The model under review builds one solid part; all positions refer to its coordinate system, in mm. Face numbers are marked on the shaded views. A direction names the side the tool comes from. Round coordinates to 2 decimals unless told otherwise and drop trailing zeros. Order: outer loops, then holes, each group sorted by start corner. A loop starts at its lowest first (then second) coordinate and runs counter-clockwise, first axis right, second up. Notation, with made-up numbers: M 80,64 L 124,64 A19 cw 124,78 Z; hole C 0.25,-28 d3. An arc over 180 degrees is marked long. Use a Markdown table: item, result. Add a question column.
1. Consider section B-B on x = 41.8. State the section outline as (y, z) points.
2. Consider section D-D on z = 17. State the section outline as (x, y) points.
3. To check wall thickness, follow probe 1 along X at (y, z) = (11.5, 12); probe 2 along Z at (x, y) = (11.5, 38); probe 3 along Z at (x, y) = (41.8, 12.6). State the ranges of each line that lie inside material, in increasing order.
4. The part is to be moulded in two halves that separate along X. For the marked faces 3, 4 and 5, say which applies: +X half, -X half, draft (parallel to the pull), parting line (faces both ways), or undercut.
5. Consider section A-A on y = 11. State the section outline as (x, z) points, then the cut area to 3 significant figures.
6. Consider section C-C on y = 23.5. State the section outline as (x, z) points.
7. Insertion check: P1, Ø1.2, axis at x = 50, z = 0, coming from the +Y side; P2, Ø2.5, axis at x = 8, z = 7.5, coming from the +Y side; P3, Ø0.8, axis at x = 41.5, z = 23.5, coming from the +Y side. Each pin has a flat end and moves straight along its axis. Give the tip position at first contact, or say it passes through.
8. For the marked faces 1 and 2, list the 3-axis set-ups (+Z, -Z, +X, -X, +Y, -Y) from which the entire face can be reached by the end or side of a thin tool; tool diameter is ignored.
from build123d import *

# Parameters (mm, degrees)
SKETCH1_W           = 50
SKETCH1_H           = 30
BOSS_EXTRUDE1_DEPTH = 5
SKETCH1_3_W         = 60
SKETCH1_3_H         = 40
SKETCH1_3_W_2       = 50
SKETCH1_3_H_2       = 30
BOSS_EXTRUDE2_DEPTH = 40
SKETCH2_R           = 4
BOSS_EXTRUDE3_DEPTH = 10
SKETCH6_R           = 0.75
CUT_EXTRUDE1_DEPTH  = 5
FILLET1_R           = 1.5
BOSS_EXTRUDE4_START = -1e-06
BOSS_EXTRUDE4_DEPTH = 35.000001
SKETCH10_R          = 0.75
CUT_EXTRUDE2_DEPTH  = 10
FILLET2_R           = 1


with BuildPart() as part:
    # Sketch1 → Boss-Extrude1 (new body)
    with BuildSketch(Plane(origin=(0, 0, 0), x_dir=(1, 0, 0), z_dir=(0, 1, 0))):
        with Locations((25, -15)):
            Rectangle(SKETCH1_W, SKETCH1_H)
    extrude(amount=BOSS_EXTRUDE1_DEPTH)

    # Sketch1<3> → Boss-Extrude2 (add)
    with BuildSketch(Plane(origin=(0, 0, 0), x_dir=(1, 0, 0), z_dir=(0, 1, 0))):
        with Locations((25, -15)):
            Rectangle(SKETCH1_3_W, SKETCH1_3_H)
        with Locations((25, -15)):
            Rectangle(SKETCH1_3_W_2, SKETCH1_3_H_2, mode=Mode.SUBTRACT)
    extrude(amount=BOSS_EXTRUDE2_DEPTH)

    # Sketch2 → Boss-Extrude3 (add)
    with BuildSketch(Plane(origin=(0, 5, 0), x_dir=(1, 0, 0), z_dir=(0, 1, 0))):
        with Locations((8.2, -6.5)):
            Circle(SKETCH2_R)
        with Locations((41.8, -23.5)):
            Circle(SKETCH2_R)
    extrude(amount=BOSS_EXTRUDE3_DEPTH)

    # Sketch6 → Cut-Extrude1 (cut)
    with BuildSketch(Plane(origin=(0, 15, 0), x_dir=(1, 0, 0), z_dir=(0, 1, 0))):
        with Locations((41.8, -23.4)):
            Circle(SKETCH6_R)
        with Locations((8.1, -6.6)):
            Circle(SKETCH6_R)
    extrude(amount=-CUT_EXTRUDE1_DEPTH, mode=Mode.SUBTRACT)

    # Fillet1
    fillet1_edges = [part.edges().sort_by_distance(p)[0] for p in [
        (4.2, 5, 6.5),
        (37.8, 5, 23.5),
    ]]
    fillet(fillet1_edges, radius=FILLET1_R)

    # Sketch9 → Boss-Extrude4 (add)
    with BuildSketch(Plane(origin=(0, 5, 0), x_dir=(1, 0, 0), z_dir=(0, 1, 0)).offset(BOSS_EXTRUDE4_START)):
        with BuildLine():
            Line((5, 0), (0, 0))
            Line((0, 0), (0, -5))
            ThreePointArc((0, -5), (3.535533906, -3.535533906), (5, 0))
        make_face()
        with BuildLine():
            Line((50, -5), (50, 0))
            Line((50, 0), (45, 0))
            ThreePointArc((45, 0), (46.464466094, -3.535533906), (50, -5))
        make_face()
        with BuildLine():
            Line((45, -30), (50, -30))
            Line((50, -30), (50, -25))
            ThreePointArc((50, -25), (46.464466094, -26.464466094), (45, -30))
        make_face()
        with BuildLine():
            Line((0, -25), (0, -30))
            Line((0, -30), (5, -30))
            ThreePointArc((5, -30), (3.535533906, -26.464466094), (0, -25))
        make_face()
    extrude(amount=BOSS_EXTRUDE4_DEPTH)

    # Sketch10 → Cut-Extrude2 (cut)
    with BuildSketch(Plane(origin=(0, 40, 0), x_dir=(1, 0, 0), z_dir=(0, 1, 0))):
        with Locations((50, -30)):
            Circle(SKETCH10_R)
        with Locations((0, -30)):
            Circle(SKETCH10_R)
        with Locations((50, 0)):
            Circle(SKETCH10_R)
        Circle(SKETCH10_R)
    extrude(amount=-CUT_EXTRUDE2_DEPTH, mode=Mode.SUBTRACT)

    # Fillet2
    fillet2_edges = [part.edges().sort_by_distance(p)[0] for p in [
        (-5, 20, -5),
        (-5, 20, 35),
        (55, 20, 35),
        (55, 20, -5),
    ]]
    fillet(fillet2_edges, radius=FILLET2_R)


solid = part.part
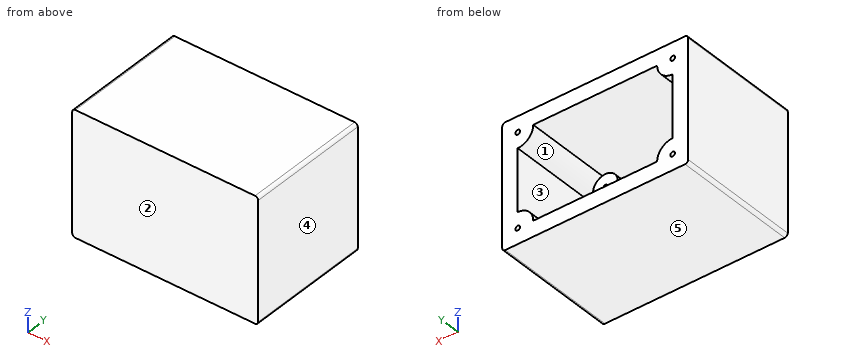
Answer block:
| question | item | result |
|---|---|---|
| 1 | outline | M 0,-5 L 40,-5 L 40,0 L 5,0 L 5,18 A1.5 cw 6.5,19.5 L 15,19.5 L 15,22.65 L 10,22.65 L 10,24.15 L 15,24.15 L 15,27.5 L 6.5,27.5 A1.5 cw 5,29 L 5,30 L 40,30 L 40,35 L 0,35 Z |
| 2 | outline | M -5,0 L 55,0 L 55,40 L 50,40 L 50,5 L 0,5 L 0,40 L -5,40 Z |
| 3 | probe 1 | -5 to 0, 50 to 55 |
| 3 | probe 2 | -5 to 0, 30 to 35 |
| 3 | probe 3 | -5 to 0, 19.5 to 22.65, 24.15 to 27.5, 30 to 35 |
| 4 | face 3 | undercut |
| 4 | face 4 | +X half |
| 4 | face 5 | draft |
| 5 | outline | M -5,-4 A1 ccw -4,-5 L 54,-5 A1 ccw 55,-4 L 55,34 A1 ccw 54,35 L -4,35 A1 ccw -5,34 Z; C 8.2,6.5 d8; C 41.8,23.5 d8; hole M 0,5 A5 cw 5,0 L 45,0 A5 cw 50,5 L 50,25 A5 cw 45,30 L 5,30 A5 cw 0,25 Z; hole C 8.1,6.6 d1.5; hole C 41.8,23.4 d1.5 |
| 5 | area | 1,070 mm^2 |
| 6 | outline | M -5,-4 A1 ccw -4,-5 L 54,-5 A1 ccw 55,-4 L 55,34 A1 ccw 54,35 L -4,35 A1 ccw -5,34 Z; hole M 0,5 A5 cw 5,0 L 45,0 A5 cw 50,5 L 50,25 A5 cw 45,30 L 5,30 A5 cw 0,25 Z |
| 7 | P1 | y = 30 |
| 7 | P2 | y = 15 |
| 7 | P3 | y = 10 |
| 8 | face 1 | +Y |
| 8 | face 2 | +Z, -Z, +X, -X, -Y |
